The listing builds one solid part. Answer for the finished solid, in the listing's coordinates (mm). A direction names the side the tool comes from. Give positions to 0.01 mm unless a question says otherwise; leave off trailing zeros. Order: outer loops, then holes, each group sorted by start corner. A loop starts at its lowest first (then second) coordinate and runs counter-clockwise, first axis right, second up. Notation, with made-up numbers: (24, 17) - (48, 17) arc R16 cw to (48, 31) - close; hole circle Ø7 at (63, -24.5). An arc over 180 degrees is marked (long way). Answer as CSV lines item,"result". Start each with the question number.
1. Flat-ended cylindrical pins translate along their axes: pin 1 (10 mm diameter, centred on y = 8, z = 21, fed in from -X); pin 2 (1 mm diameter, centred on x = -12.5, z = -9.5, fed in from +Y); pin 3 (4.5 mm diameter, centred on y = 14.5, z = 0, fed in from +X). Find the tip coordinate at first contact, or state that the pin passes through.
2. Section C-C on y = 14.5 is taken. Give the vertices of the cut face in (x, z).
3. Which of the six approach directions +Z, -Z, +X, -X, +Y, -Y give full straight-line access (tool end or side, diameter ignored) to faces 1 (the cylindrical face through (-3.252, 14.451, 14.643)), 2 (the cylindrical face through (-5.961, 0.986, 26.846)), 3 (the flat face through (12.1, 2, 22.3)), 4 (the cylindrical face through (-1.998, 14.588, -8.157))?
4. Section D-D on z = -8.5 is taken. Give the vertices of the cut face in (x, y), and give its area (3 significant figures).
5. Section A-A on z = 0 is taken. Give the vertices of the cut face in (x, y), and give its area (3 significant figures).
6. Consider line 1 along Y through (x, z) = (-24, 12.5); line 2 along Y through (x, z) = (10.25, 0); line 3 along Z through (x, y) = (0, 6). Determine where each line is inside the solid, lowest interval first. Write a range as [from, to].
7. Section B-B on x = 0 is taken. Give the vertices of the cut face in (y, z).
8. Determine the mould class of faces 5 (the flat face through (12, 11, 12)), 6 (the cylindrical face through (-5.961, 9.986, 26.846)), 7 (the cylindrical face through (8.156, 14.588, -1.998)), 8 (the flat face through (0, 0, 6)) for opening direction Y: +Y half, -Y half, draft (parallel to the pull), parting line (faces both ways), or undercut.
from build123d import *

# Parameters (mm, degrees)
SKETCH1_R           = 27.5
BOSS_EXTRUDE1_DEPTH = 2
SKETCH2_R           = 25
BOSS_EXTRUDE2_DEPTH = 7
SKETCH3_R           = 27.5
BOSS_EXTRUDE3_DEPTH = 2
SKETCH4_R           = 15
BOSS_EXTRUDE4_DEPTH = 7
SKETCH5_R           = 2.5
CUT_EXTRUDE1_DEPTH  = 19
SKETCH6_R           = 2
CUT_EXTRUDE2_DEPTH  = 28.5
CIRPATTERN1_COUNT   = 2
CIRPATTERN1_ANGLE   = 90


with BuildPart() as part:
    # Sketch1 → Boss-Extrude1 (new body)
    with BuildSketch(Plane(origin=(0, 0, 0), x_dir=(1, 0, 0), z_dir=(0, 1, 0))):
        Circle(SKETCH1_R)
    extrude(amount=BOSS_EXTRUDE1_DEPTH)

    # Sketch2 → Boss-Extrude2 (add)
    with BuildSketch(Plane(origin=(0, 2, 0), x_dir=(1, 0, 0), z_dir=(0, 1, 0))):
        Circle(SKETCH2_R)
    extrude(amount=BOSS_EXTRUDE2_DEPTH)

    # Sketch3 → Boss-Extrude3 (add)
    with BuildSketch(Plane(origin=(0, 9, 0), x_dir=(1, 0, 0), z_dir=(0, 1, 0))):
        Circle(SKETCH3_R)
    extrude(amount=BOSS_EXTRUDE3_DEPTH)

    # Sketch4 → Boss-Extrude4 (add)
    with BuildSketch(Plane(origin=(0, 11, 0), x_dir=(1, 0, 0), z_dir=(0, 1, 0))):
        Circle(SKETCH4_R)
    extrude(amount=BOSS_EXTRUDE4_DEPTH)

    # Sketch5 → Cut-Extrude1 (cut, through all)
    with BuildSketch(Plane(origin=(0, 18, 0), x_dir=(1, 0, 0), z_dir=(0, 1, 0))):
        Circle(SKETCH5_R)
    extrude(amount=-CUT_EXTRUDE1_DEPTH, mode=Mode.SUBTRACT)

    # Sketch6 → Cut-Extrude2 (cut, through all)
    with BuildSketch(Plane.XY):
        with Locations((0, 14.5)):
            Circle(SKETCH6_R)
    cut_extrude2 = extrude(amount=-CUT_EXTRUDE2_DEPTH, mode=Mode.SUBTRACT)

    # CirPattern1: Cut-Extrude2 ×2 about axis
    cirpattern1_axis = Axis((0, 18, 0), (0, -1, 0))
    for i in range(1, CIRPATTERN1_COUNT):
        add(cut_extrude2.rotate(cirpattern1_axis, i * CIRPATTERN1_ANGLE / (CIRPATTERN1_COUNT - 1)), mode=Mode.SUBTRACT)


solid = part.part
Checks:
1,pin 1,"stops at x = -22.29"
1,pin 2,"stops at y = 11"
1,pin 3,"stops at x = 15"
2,outline,"(-2, -14.87) - (-2, -1.5) arc R2.5 cw to (1.5, 2) - (14.87, 2) arc R15 ccw (long way) to start; (2, -14.87) arc R15 ccw to (14.87, -2) - (2, -2) - close"
3,face 1,"+Y"
3,face 2,"+Y, -Y"
3,face 3,"none"
3,face 4,"-Z"
4,outline,"(-26.15, 0) - (26.15, 0) - (26.15, 2) - (23.51, 2) - (23.51, 9) - (26.15, 9) - (26.15, 11) - (12.36, 11) - (12.36, 18) - (-12.36, 18) - (-12.36, 11) - (-26.15, 11) - (-26.15, 9) - (-23.51, 9) - (-23.51, 2) - (-26.15, 2) - close; hole circle Ø4 at (0, 14.5)"
4,area,"699 mm²"
5,outline,"(-27.5, 0) - (-2.5, 0) - (-2.5, 18) - (-15, 18) - (-15, 11) - (-27.5, 11) - (-27.5, 9) - (-25, 9) - (-25, 2) - (-27.5, 2) - close; (2.5, 0) - (27.5, 0) - (27.5, 2) - (25, 2) - (25, 9) - (27.5, 9) - (27.5, 11) - (15, 11) - (15, 12.5) - (2.5, 12.5) - close; (2.5, 16.5) - (15, 16.5) - (15, 18) - (2.5, 18) - close"
5,area,"640 mm²"
6,line 1,"y = [0, 2], [9, 11]"
6,line 2,"y = [0, 12.5], [16.5, 18]"
6,line 3,"z = [-25, -2.5], [2.5, 25]"
7,outline,"(0, -27.5) - (2, -27.5) - (2, -25) - (9, -25) - (9, -27.5) - (11, -27.5) - (11, -15) - (12.5, -15) - (12.5, -2.5) - (0, -2.5) - close; (0, 2.5) - (18, 2.5) - (18, 15) - (11, 15) - (11, 27.5) - (9, 27.5) - (9, 25) - (2, 25) - (2, 27.5) - (0, 27.5) - close; (16.5, -15) - (18, -15) - (18, -2.5) - (16.5, -2.5) - close"
8,face 5,"+Y half"
8,face 6,"draft"
8,face 7,"undercut"
8,face 8,"-Y half"
